Could you check a few things on this model? Use its own coordinates, in mm. Give positions to 0.01 mm unless a question says otherwise; leave off trailing zeros. Order: outer loops, then holes, each group sorted by start corner. A loop starts at its lowest first (then second) coordinate and runs counter-clockwise, first axis right, second up. Notation, with made-up numbers: (0, 38.25) - (50, 38.25) arc R16 cw to (50, 51.25) - close; hole circle Ø9 at (33, -27.75). An arc over 180 degrees is marked (long way). Put each result on its own line as item: value.
from build123d import *

# Parameters (mm, degrees)
SKETCH_R      = 162.5
PAD_DEPTH     = 200
SKETCH001_R   = 20.44
HOLE_DEPTH    = 337.501
SKETCH002_R   = 20.44
HOLE001_DEPTH = 337.501


with BuildPart() as part:
    # Sketch → Pad (new body)
    with BuildSketch(Plane.XY):
        Circle(SKETCH_R)
    extrude(amount=PAD_DEPTH)

    # Sketch001 → Hole (cut, through all)
    with BuildSketch(Plane.YZ.offset(175)):
        with Locations((0, 199.9)):
            Circle(SKETCH001_R)
    extrude(amount=-HOLE_DEPTH, mode=Mode.SUBTRACT)

    # Sketch002 → Hole001 (cut, through all)
    with BuildSketch(Plane.XZ.offset(175)):
        with Locations((0, 199.9)):
            Circle(SKETCH002_R)
    extrude(amount=-HOLE001_DEPTH, mode=Mode.SUBTRACT)


solid = part.part
1) We'd pull the mould along Y, two halves only. Please class faces 1 (the cylindrical face through (155, 48.8, 98.6)), 2 (the cylindrical face through (-80.113, -0.451, 179.465)), 3 (the flat face through (74, 76, 200)): pulls with the +Y half, pulls with the -Y half, needs draft (parallel to the pull), parting line crosses it, or undercut.
Filled in:
face 1: parting line crosses it
face 2: undercut
face 3: needs draft
2) I'm going to push flat-ended pins straight in: pin 1 (2 mm diameter, centred on x = -35.5, y = -50, fed in from -Z); pin 2 (2 mm diameter, centred on y = 110.5, z = 165, fed in from -X); pin 3 (1 mm diameter, centred on x = 112.5, z = 89, fed in from +Y); pin 4 (8 mm diameter, centred on x = -5, y = 27.5, fed in from +Z). Where does each tip first touch, or does it pass through?
Filled in:
pin 1: stops at z = 0
pin 2: stops at x = -120.07
pin 3: stops at y = 117.74
pin 4: stops at z = 181.55
3) Suppose I cut it at B-B, the plane z = 161.5. List the corners of the cut face in (x, y) for me.
Filled in:
outline: circle Ø325 at (0, 0)
4) Suppose I cut it at A-A, the plane y = 44. List the corners of the cut face in (x, z) for me, and give its area (3 significant figures).
Filled in:
outline: (-156.43, 0) - (156.43, 0) - (156.43, 200) - (20.44, 200) arc R20.44 cw (long way) to (-20.44, 200) - (-156.43, 200) - close
area: 61,900 mm^2
5) If I drill on line 1 (Y direction, x = -132, z = 187); line 2 (Y direction, x = 4, z = 9.5); line 3 (X direction, y = -5.5, z = 40), over which ranges is the centre line in solid material (lowest first)? Write a range as [from, to].
Filled in:
line 1: y = [-94.77, -15.86], [15.86, 94.77]
line 2: y = [-162.45, 162.45]
line 3: x = [-162.41, 162.41]
6) Suppose I cut it at C-C, the plane x = 104. List the corners of the cut face in (y, z) for me.
Filled in:
outline: (-124.86, 0) - (124.86, 0) - (124.86, 200) - (20.44, 200) arc R20.44 cw (long way) to (-20.44, 200) - (-124.86, 200) - close
